Design review of the part shown in the three views and the two pictorial views. Dimensions are in mm from the part's minimum x, y and z. A direction names the side the tool comes from. Round coordinates to 2 decimals unless told otherwise and drop trailing zeros. Loops run counter-clockwise (first coordinate to the right, second up) from the corner with the lowest first, then second, coordinate; pieces in that order, holes last. Notation, with made-up numbers: M 12.25,51 L 61.25,51 A19 cw 61.25,83 Z; hole C -20.5,39.5 d4. An arc over 180 degrees is marked long. One line per question, with ' | ' between items.
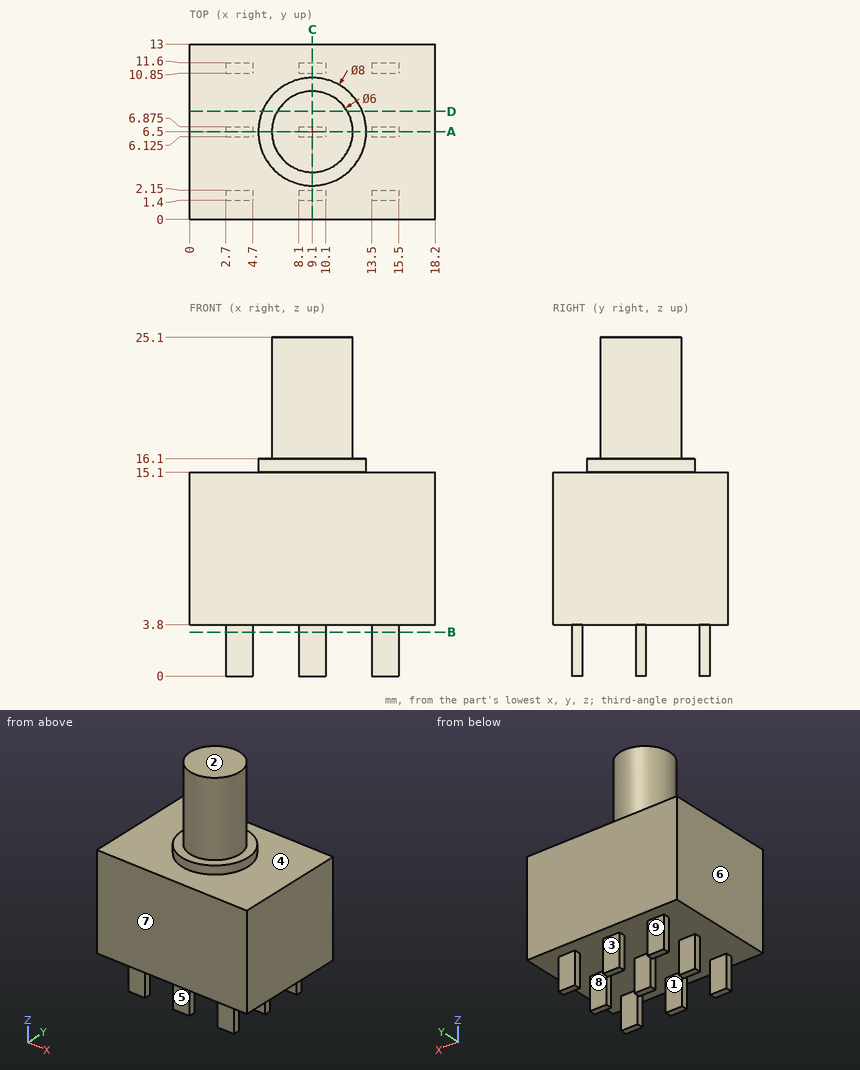
1) Insertion check: P1, Ø1, axis at x = 4, z = 2, coming from the +Y side; P2, Ø0.6, axis at x = 3.5, z = 2, coming from the -Y side; P3, Ø0.6, axis at y = 6.5, z = 1.5, coming from the +X side; P4, Ø5, axis at x = 2, z = 20.5, coming from the +Y side. Each pin has a flat end and moves straight along its axis. Give the tip position at first contact, or say it passes through.
Output values:
P1: stops at y = 11.6 | P2: stops at y = 1.4 | P3: stops at x = 15.5 | P4: passes through
2) For line 1 (Z direction, x = 3.25, y = 6); line 2 (Z direction, x = 3, y = 2); line 3 (X direction, y = 8, z = 17.5), list the stretches that pass through material, from the lowest coordinate up.
Output values:
line 1: z = 3.8 to 15.1 | line 2: z = 0 to 15.1 | line 3: x = 6.5 to 11.7
3) Machinability: for the marked faces 1, 2, 3, 4 and 5, which of the approach directions +Z, -Z, +X, -X, +Y, -Y give a long, thin tool a straight path to every point of the face, cutting with its end or side? Answer none if there is none.
Output values:
face 1: -Z, +X, -X | face 2: +Z, +X, -X, +Y, -Y | face 3: -Z, +X, -X, +Y | face 4: +Z | face 5: -Z, +X, -X, -Y
4) Add section B-B on z = 3.25. State how many separate pieces and enclosed holes the cut face has, then the cut area to 3 significant figures.
Output values:
separate pieces: 9 | enclosed holes: 0 | area: 13.5 mm²
5) Add section D-D on y = 8. State the section outline as (x, z) points.
Output values:
outline: M 0,3.8 L 18.2,3.8 L 18.2,15.1 L 12.81,15.1 L 12.81,16.1 L 11.7,16.1 L 11.7,25.1 L 6.5,25.1 L 6.5,16.1 L 5.39,16.1 L 5.39,15.1 L 0,15.1 Z
6) Add section A-A on y = 6.5. State the section outline as (x, z) points.
Output values:
outline: M 0,3.8 L 2.7,3.8 L 2.7,0 L 4.7,0 L 4.7,3.8 L 8.1,3.8 L 8.1,0 L 10.1,0 L 10.1,3.8 L 13.5,3.8 L 13.5,0 L 15.5,0 L 15.5,3.8 L 18.2,3.8 L 18.2,15.1 L 13.1,15.1 L 13.1,16.1 L 12.1,16.1 L 12.1,25.1 L 6.1,25.1 L 6.1,16.1 L 5.1,16.1 L 5.1,15.1 L 0,15.1 Z
7) Add section C-C on x = 9.1. State the section outline as (y, z) points (3 decimals), then the cut area to 3 significant figures.
Output values:
outline: M 0,3.8 L 1.4,3.8 L 1.4,0 L 2.15,0 L 2.15,3.8 L 6.125,3.8 L 6.125,0 L 6.875,0 L 6.875,3.8 L 10.85,3.8 L 10.85,0 L 11.6,0 L 11.6,3.8 L 13,3.8 L 13,15.1 L 10.5,15.1 L 10.5,16.1 L 9.5,16.1 L 9.5,25.1 L 3.5,25.1 L 3.5,16.1 L 2.5,16.1 L 2.5,15.1 L 0,15.1 Z | area: 217 mm²
8) Mouldability with a two-part tool opening along Y and no side actions: class the marked faces 6, 7, 8 and 9 as +Y half, -Y half, draft (parallel to the pull), parting line (faces both ways), or undercut.
Output values:
face 6: draft | face 7: -Y half | face 8: undercut | face 9: +Y half
